The drawing under review shows one solid part. Ordinate dimensions are in mm from its lowest x, y, z. A direction names the side the tool comes from. Coordinates: 2 decimals unless noted, no trailing zeros. Write each loop counter-clockwise with the first axis right and the second up, starting at its lowest first coordinate (ties: lowest second). Pieces come first, ordered by that corner, then holes.
1) Add section D-D, the plane x = 33. State the section outline as (y, z) points, then the cut area to 3 significant figures.
2) For P1, Ø6, axis at x = 21.5, z = 5, coming from the +Y side; P2, Ø1.5, axis at x = 13.5, y = 1.5, coming from the +Z side; P3, Ø1, axis at y = 2.5, z = 9.5, coming from the -X side; P4, Ø10, axis at x = 30, z = 7, coming from the -Y side, all flat-tipped, find the tip position at first contact; note any pin that passes through.
3) Machinability: for the marked faces 1 and 2, which of the approach directions +Z, -Z, +X, -X, +Y, -Y give a long, thin tool a straight path to every point of the face, cutting with its end or side? Answer none if there is none.
4) For line 1 (Z direction, x = 20.4, y = 1.1); line 2 (Y direction, x = 26, z = 38), list the stretches that pass through material, from the lowest coordinate up.
5) Mouldability with a two-part tool opening along Z and no side actions: class the marked faces 3, 4 and 5 as released by +Z, released by -Z, zero draft, split by the parting line, or undercut.
6) Add section B-B, the plane x = 20.4. State the section outline as (y, z) points, then the cut area to 3 significant figures.
7) Add section C-C, the plane x = 9. State the section outline as (y, z) points, then the cut area to 3 significant figures.
8) Add section A-A, the plane y = 2.3. State the section outline as (x, z) points.
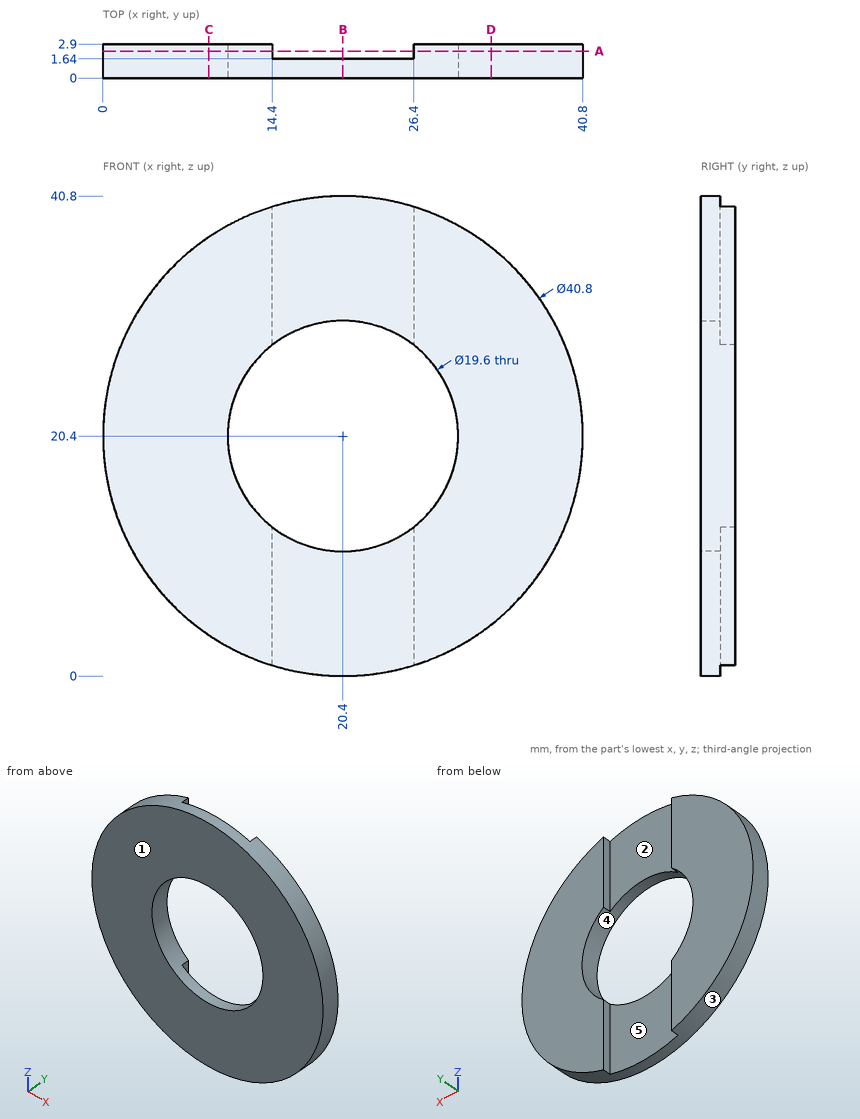
Geometry results:
1. outline: (0, 4.36) - (2.9, 4.36) - (2.9, 36.44) - (0, 36.44) - close
1. area: 93.1 mm2
2. P1: stops at y = 1.64
2. P2: stops at z = 39.85
2. P3: stops at x = 2.85
2. P4: stops at y = 0
3. face 1: +Z, -Z, +X, -X, -Y
3. face 2: +Z, -Z, +Y
4. line 1: z = 0 to 10.6, 30.2 to 40.8
4. line 2: y = 0 to 1.64
5. face 3: split by the parting line
5. face 4: undercut
5. face 5: zero draft
6. outline: (0, 0) - (1.64, 0) - (1.64, 10.6) - (0, 10.6) - close; (0, 30.2) - (1.64, 30.2) - (1.64, 40.8) - (0, 40.8) - close
6. area: 34.8 mm2
7. outline: (0, 3.48) - (2.9, 3.48) - (2.9, 37.32) - (0, 37.32) - close
7. area: 98.1 mm2
8. outline: (14.4, 0.9) - (14.4, 12.65) arc R9.8 cw to (14.4, 28.15) - (14.4, 39.9) arc R20.4 ccw to start; (26.4, 0.9) arc R20.4 ccw to (26.4, 39.9) - (26.4, 28.15) arc R9.8 cw to (26.4, 12.65) - close
